Build history of the part. All positions in model axes, mm. A direction names the side the tool comes from. Give positions to 0.01 mm unless a question says otherwise; leave off trailing zeros. Write each loop counter-clockwise with the first axis right and the second up, starting at its lowest first coordinate (ties: lowest second). Pieces come first, ordered by that corner, then holes. Notation, with made-up numbers: (4, -20.5) -> (55, -20.5) arc R18 ccw to (55, -13.5) -> close; hole circle Ø1 at (54.25, 79). An arc over 180 degrees is marked (long way). Put each result on its own line as item: value. Start each with the question number.
Item 1: Drill centre lines: line 1 along Y through (x, z) = (-3, 122.5); line 2 along Y through (x, z) = (0.25, 37); line 3 along Z through (x, y) = (0, -3.5). Where is each one in solid material? Low to high.
Item 2: Slice it at A-A, the plane y = 0. List the corners of the cut face in (x, z) (3 decimals).
Item 3: Tool access for faces 1 (the flat face through (0, 0, 0)), 2 (the cylindrical face through (4.967, -1.564, 111.429)): list every direction of +Z, -Z, +X, -X, +Y, -Y with a clear straight run to the whole face (end or side of a thin tool).
Item 4: Slice it at C-C, the plane z = 26. List the corners of the cut face in (x, y).
Item 5: Flat gauge pins, fed straight in: pin 1 Ø10 at (x, y) = (-5, -6.5) entering from +Z; pin 2 Ø1.5 at (x, z) = (0, 62.5) entering from +Y; pin 3 Ø1.5 at (y, z) = (-5, 79) entering from -X; pin 4 Ø8 at (y, z) = (5.5, 74) entering from -X. Where does each tip first touch, or does it go through?
Item 6: Slice it at D-D, the plane z = 119.5. List the corners of the cut face in (x, y).
```python
from build123d import *


# Not quite as in the source:
# - a fillet or chamfer that OpenCascade refuses, or shapes differently, is made with other operations: its cross-section is extruded or revolved along the edge and cut away or added


with BuildPart() as f1:
    # F0 (on Front) → F1 (revolve)
    with BuildSketch(Plane.XZ):
        Polygon((0, 113.175), (0, 0), (3.683, 0), (3.683, 110), (5.207, 110), (5.207, 113.175), align=None)
    revolve(axis=Axis((0, 0, 56.5875), (0, 0, -1)))

    # F2: fillet of radius 2.54 on 1 edges, made by hand

    # F2_s1 → F2_t2 (revolve)
    with BuildSketch(Plane.XZ):
        with BuildLine():
            ThreePointArc((3.683, 107.672051547), (4.0978835326, 109.063266843), (5.207, 110))
            Line((5.207, 110), (3.683, 110))
            Line((3.683, 110), (3.683, 107.672051547))
        make_face()
    revolve(axis=Axis((0, 0, 110), (0, 0, -1)))

    # F3 (on Front) → F4 (revolve)
    with BuildSketch(Plane.XZ):
        with BuildLine():
            ThreePointArc((0, 111.27), (6.7351920908, 114.0598079092), (9.525, 120.795))
            ThreePointArc((9.525, 120.795), (6.7351920908, 127.5301920908), (0, 130.32))
            Line((0, 130.32), (0, 111.27))
        make_face()
    revolve(axis=Axis((0, 0, 120.795), (0, 0, -1)))


solid = f1.part
```
Values follow:
1. line 1: -8.88 to 8.88
1. line 2: -3.67 to 3.67
1. line 3: 0 to 129.65
2. outline: (-5.207, 110) arc R2.54 cw to (-3.683, 107.672) -> (-3.683, 0) -> (3.683, 0) -> (3.683, 107.672) arc R2.54 cw to (5.207, 110) -> (5.207, 112.819) arc R9.525 ccw (long way) to (-5.207, 112.819) -> close
3. face 1: -Z, +X, -X, +Y, -Y
3. face 2: -Z
4. outline: circle Ø7.37 at (0, 0)
5. pin 1: z = 129.77
5. pin 2: y = 3.68
5. pin 3: through
5. pin 4: x = -3.36
6. outline: circle Ø18.87 at (0, 0)
